Could you check a few things on this model? Use its own coordinates, in mm. A direction names the side the tool comes from. Coordinates: 2 decimals unless noted, no trailing zeros. Write each loop counter-clockwise with the first axis right and the second up, starting at its lowest first coordinate (ties: lowest second). Pieces come first, ordered by that corner, then holes.
Item 1: I want a section at C-C on y = 12.5. Please give me the cut outline in (x, z).
Item 2: I want a section at A-A on x = -122.75. Please give me the cut outline in (y, z).
Item 3: Thinking about a two-plate mould opening in Y: for faces 1 (the cylindrical face through (-129.873, 19.72, -5.75)), 2 (the flat face through (-125, 0, -6)), 3 (the flat face through (-122, 31.5, -6)), which applies, +Y half, -Y half, draft (parallel to the pull), parting line (faces both ways), or undercut?
Item 4: Which directions (+Z, -Z, +X, -X, +Y, -Y) give clear straight access to the entire face, cutting with the end or side of a thin tool? Please do faces 4 (the cylindrical face through (-124.875, 33.472, -5.599)), 5 (the flat face through (-125, 40, -6)).
Item 5: I want a section at D-D on z = 3.75. Please give me the cut outline in (x, y), then the cut area to 3 significant figures.
Item 6: If I drill on probe 1 along Y at (x, z) = (-121.5, -6.5); probe 2 along Z at (x, y) = (-125, 6.5); probe 3 along X at (y, z) = (18, -1.25), over which ranges is the centre line in solid material (lowest first)?
Item 7: For P1, Ø3, axis at x = -126.5, y = 19.5, coming from the -Z side, with a flat end and sliding along its axis, tell me the tip position at first contact or that it passes through.
Item 8: I want a section at B-B on z = -1. Please give me the cut outline in (x, y).
from build123d import *

# Parameters (mm, degrees)
BOSS_EXTRUDE1_DEPTH = 40
CUT_EXTRUDE4_DEPTH  = 4


with BuildPart() as part:
    # Sketch1 → Boss-Extrude1 (new body)
    with BuildSketch(Plane(origin=(0, 0, 0), x_dir=(1, 0, 0), z_dir=(0, 1, 0))):
        with BuildLine():
            ThreePointArc((-129.505310752, 11.330246557), (-129.876268806, 5.670520357), (-130, 0))
            ThreePointArc((-130, 0), (-125, -5), (-120, 0))
            ThreePointArc((-120, 0), (-119.88578659, 5.234326484), (-119.543363771, 10.45868913))
            ThreePointArc((-119.543363771, 10.45868913), (-124.088558548, 15.875441334), (-129.505310752, 11.330246557))
        make_face()
    extrude(amount=BOSS_EXTRUDE1_DEPTH)

    # Sketch2 → Cut-Extrude4 (cut)
    with BuildSketch(Plane(origin=(0, 31.5, 0), x_dir=(1, 0, 0), z_dir=(0, 1, 0))):
        with BuildLine():
            ThreePointArc((-123.989026242, 15.865729465), (-124.881027698, 5.452423421), (-124.9, -4.9989999))
            ThreePointArc((-124.9, -4.9989999), (-121.429285786, -3.5), (-120, 0))
            ThreePointArc((-120, 0), (-119.88578659, 5.234326484), (-119.543363771, 10.45868913))
            ThreePointArc((-119.543363771, 10.45868913), (-120.662165593, 14.069941037), (-123.989026242, 15.865729465))
        make_face()
    extrude(amount=CUT_EXTRUDE4_DEPTH, mode=Mode.SUBTRACT)


solid = part.part
Response values:
1. outline: (-130, 0) arc R130 ccw to (-129.51, -11.33) arc R5 ccw to (-119.54, -10.46) arc R120 cw to (-120, 0) arc R5 ccw to start
2. outline: (0, -15.57) - (31.5, -15.57) - (31.5, 4.47) - (0, 4.47) - close; (35.5, -15.57) - (40, -15.57) - (40, 4.47) - (35.5, 4.47) - close
3. face 1: draft
3. face 2: -Y half
3. face 3: undercut
4. face 4: +X
4. face 5: +Z, -Z, +X, -X, +Y
5. outline: (-128.31, 0) - (-121.69, 0) - (-121.69, 31.5) - (-124.94, 31.5) - (-124.94, 35.5) - (-121.69, 35.5) - (-121.69, 40) - (-128.31, 40) - close
5. area: 252 mm2
6. probe 1: y = 0 to 31.5, 35.5 to 40
6. probe 2: z = -15.87 to 5
6. probe 3: x = -129.99 to -119.99
7. P1: stops at z = -15.87
8. outline: (-130, 0) - (-120, 0) - (-120, 31.5) - (-125, 31.5) - (-125, 35.5) - (-120, 35.5) - (-120, 40) - (-130, 40) - close
